Input: dimensioned drawing with shaded views. Units: mm. Origin: part minimum x, y, z. A direction names the side the tool comes from. Coordinates: 2 decimals unless noted, no trailing zeros. Loops run counter-clockwise (first coordinate to the right, second up) from the corner with the lowest first, then second, coordinate; pieces in that order, holes last. Notation, with made-up numbers: (69, 33.5) - (94, 33.5) arc R27 ccw to (94, 68.5) - close; hole circle Ø1 at (81, 62.5). An arc over 180 degrees is marked (long way). Use one line per item in the form item = value. Start each with the question number.
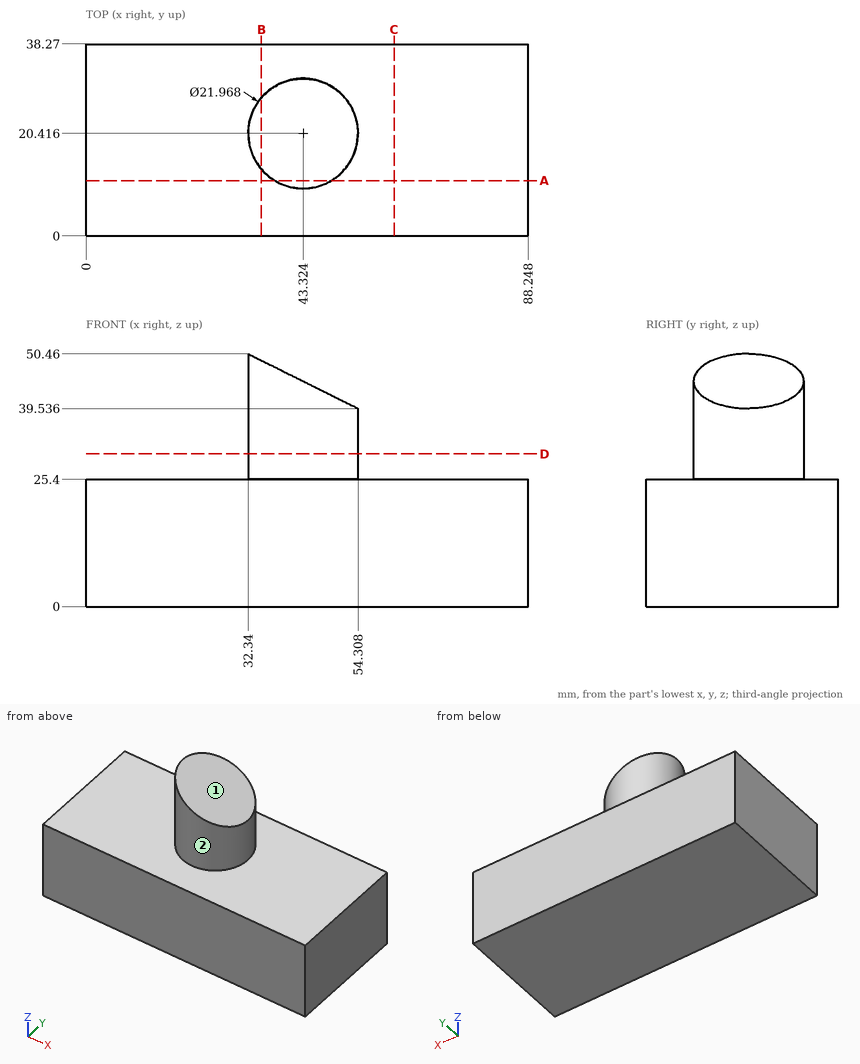
(1) Cut plane C-C, the plane x = 61.5. Output: boundary loops of the cut face in (y, z), plus the area to 3 significant figures.
(2) Material intervals for line 1 (Z direction, x = 14, y = 10); line 2 (Z direction, x = 44, y = 11.5); line 3 (X direction, y = 24, z = 45.5) (1 decimal), sorted ascending.
(3) Access query for the marked faces 1 and 2. Directions: +Z, -Z, +X, -X, +Y, -Y. A direction counts if a zero-diameter tool reaches every point of the face in a straight line with its end or side. Return the directions, or none.
(4) Cut plane B-B, the plane x = 35. Output: boundary loops of the cut face in (y, z), plus the area to 3 significant figures.
(5) Cut plane A-A, the plane y = 11. Output: boundary loops of the cut face in (x, z) (1 decimal).
(6) Contact query for flat-ended pins moving along their axis: pin 1 (4 mm diameter, centred on x = 79, y = 34.5, fed in from -Z); pin 2 (10 mm diameter, centred on x = 61, z = 36.5, fed in from +Y); pin 3 (1.5 mm diameter, centred on y = 18, z = 31, fed in from -X). Output: stop coordinate, or through.
(7) Cut plane D-D, the plane z = 30.5. Output: boundary loops of the cut face in (x, y) (1 decimal).
Recorded:
q1.outline = (0, 0) - (38.27, 0) - (38.27, 25.4) - (0, 25.4) - close
q1.area = 972 mm²
q2.line_1 = 0 to 25.4
q2.line_2 = 0 to 44.66
q2.line_3 = 32.9 to 42.3
q3.face_1 = +Z, +X, +Y, -Y
q3.face_2 = +Z
q4.outline = (0, 0) - (38.27, 0) - (38.27, 25.4) - (27.58, 25.4) - (27.58, 49.14) - (13.25, 49.14) - (13.25, 25.4) - (0, 25.4) - close
q4.area = 1,310 mm²
q5.outline = (0, 0) - (88.2, 0) - (88.2, 25.4) - (49, 25.4) - (49, 42.2) - (37.7, 47.8) - (37.7, 25.4) - (0, 25.4) - close
q6.pin_1 = 0
q6.pin_2 = through
q6.pin_3 = 32.47
q7.outline = circle Ø22 at (43.3, 20.4)
